from build123d import *

# Parameters (mm, degrees)
SKETCH_1_W             = 30
SKETCH_1_H             = 30
EXTRUDE_1_DEPTH        = 30
CUT_EXTRUDE_1_DEPTH    = 52.961524227
HOLE_WIZARD_M6_1_D     = 5
HOLE_WIZARD_M6_1_DEPTH = 15
HOLE_WIZARD_M6_1_TIP   = 1.502151548


with BuildPart() as part:
    # 草图1 → 凸台-拉伸1 (new body)
    with BuildSketch(Plane.XY):
        with Locations((15, 15)):
            Rectangle(SKETCH_1_W, SKETCH_1_H)
    extrude(amount=EXTRUDE_1_DEPTH)

    # 草图2 → 切除-拉伸1 (cut, through all)
    with BuildSketch(Plane.XY.offset(30)):
        Polygon((5, 0), (11, 2.485281374), (11, 4), (19, 4), (19, 2.485281374), (25, 0), align=None)
    extrude(amount=-CUT_EXTRUDE_1_DEPTH, mode=Mode.SUBTRACT)

    # M6 螺纹孔1
    with Locations(Plane(origin=(0, 30, 0), x_dir=(1, 0, 0), z_dir=(0, 1, 0))):
        with Locations((15, -15)):
            Hole(HOLE_WIZARD_M6_1_D / 2, depth=HOLE_WIZARD_M6_1_DEPTH)
            with Locations((0, 0, -(HOLE_WIZARD_M6_1_DEPTH + HOLE_WIZARD_M6_1_TIP / 2))):  # 118° drill point
                Cone(0, HOLE_WIZARD_M6_1_D / 2, HOLE_WIZARD_M6_1_TIP, mode=Mode.SUBTRACT)


solid = part.part
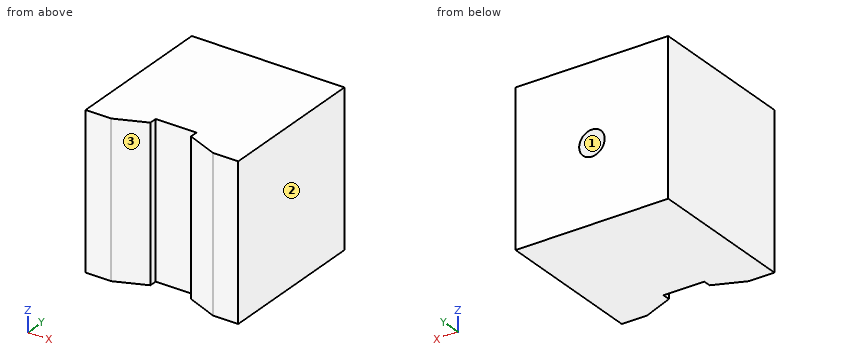
Design review of the part built by this model. Coordinates are the model's own, in mm. Face numbers are marked on the shaded views. A direction names the side the tool comes from. Give positions to 0.01 mm unless a question says otherwise; leave off trailing zeros. Loops run counter-clockwise (first coordinate to the right, second up) from the corner with the lowest first, then second, coordinate; pieces in that order, holes last. Notation, with made-up numbers: M 89.25,-35 L 146.25,-35 A28 ccw 146.25,0 Z; hole C -39,32.25 d9. An arc over 180 degrees is marked long. Write item = value, one per line.
Q1. For the marked faces 1, 2 and 3, list the 3-axis set-ups (+Z, -Z, +X, -X, +Y, -Y) from which the entire face can be reached by the end or side of a thin tool; tool diameter is ignored.
Output values:
face_1 = +Y
face_2 = +Z, -Z, +X, +Y, -Y
face_3 = +Z, -Z, -Y
Q2. We need section B-B (z = 19). Give the boundary of the cut face in (x, y), plus the area to 3 significant figures.
Output values:
outline = M 0,0 L 5,0 L 11,2.49 L 11,4 L 19,4 L 19,2.49 L 25,0 L 30,0 L 30,30 L 0,30 Z
area = 853 mm^2
Q3. Insertion check: pin 1 (5 mm diameter, centred on x = 17, z = 12.5, fed in from -Y); pin 2 (6.5 mm diameter, centred on x = 15, z = 15, fed in from -Y); pin 3 (12 mm diameter, centred on x = 12, z = 24, fed in from -Y). Each pin has a flat end and moves straight along its axis. Give the tip position at first contact, or say it passes through.
Output values:
pin_1 = 2.28
pin_2 = 4
pin_3 = 0.41
Q4. To check wall thickness, follow line 1 (Z direction, x = 15, y = 19.25); line 2 (Y direction, x = 16, z = 5.5). State the ranges of each line that lie inside material, in increasing order. Write a range as [from, to].
Output values:
line_1 = [0, 12.5], [17.5, 30]
line_2 = [4, 30]
Q5. We need section C-C (x = 8). Give the boundary of the cut face in (y, z), plus the area to 3 significant figures.
Output values:
outline = M 1.24,0 L 30,0 L 30,30 L 1.24,30 Z
area = 863 mm^2
Q6. We need section A-A (y = 22). Give the boundary of the cut face in (x, z), plus the area to 3 significant figures.
Output values:
outline = M 0,0 L 30,0 L 30,30 L 0,30 Z; hole C 15,15 d5
area = 880 mm^2
